The listing builds one solid part. Answer for the finished solid, in the listing's coordinates (mm). A direction names the side the tool comes from. Give positions to 0.01 mm unless a question says otherwise; leave off trailing zeros. Order: outer loops, then holes, each group sorted by start corner. A loop starts at its lowest first (then second) coordinate and runs counter-clockwise, first axis right, second up. Notation, with made-up numbers: (13.25, 38.25) - (63.25, 38.25) arc R8 cw to (63.25, 44.25) - close; hole circle Ø1 at (44, 68.5). An arc over 180 degrees is marked (long way). Answer in a Markdown table with one row per item.
from build123d import *

# Parameters (mm, degrees)
F0_R     = 25.2
F0_W     = 100
F0_H     = 15
F1_DEPTH = 15
F2_R     = 30
F5_DEPTH = 5


with BuildPart() as f1:
    # F0 (on Top) → F1 (new body)
    with BuildSketch(Plane.XY):
        with BuildLine():
            Line((-50, -85), (50, -85))
            Line((50, -85), (50, 40))
            Line((50, 40), (29.85, 40))
            ThreePointArc((29.85, 40), (0, 10.15), (-29.85, 40))
            Line((-29.85, 40), (-50, 40))
            Line((-50, 40), (-50, -85))
        make_face()
        with Locations((0, -45.2)):
            Circle(F0_R, mode=Mode.SUBTRACT)
        with BuildLine():
            Line((29.85, 40), (50, 40))
            Line((50, 40), (50, 70))
            Line((50, 70), (-50, 70))
            Line((-50, 70), (-50, 40))
            Line((-50, 40), (-29.85, 40))
            ThreePointArc((-29.85, 40), (0, 69.85), (29.85, 40))
        make_face()
        with Locations((0, 77.5)):
            Rectangle(F0_W, F0_H)
    extrude(amount=F1_DEPTH)

    # F2
    f2_edges = [f1.edges().sort_by_distance(p)[0] for p in [
        (-50, 85, 7.5),
        (50, 85, 7.5),
        (-50, -85, 7.5),
        (50, -85, 7.5),
    ]]
    fillet(f2_edges, radius=F2_R)

    # F4 (on face) → F5 (cut)
    with BuildSketch(Plane.XY.offset(15)):
        with BuildLine():
            ThreePointArc((45, 55), (37.67767, 72.67767), (20, 80))
            Line((20, 80), (-20, 80))
            ThreePointArc((-20, 80), (-37.67767, 72.67767), (-45, 55))
            Line((-45, 55), (-45, -55))
            ThreePointArc((-45, -55), (-37.67767, -72.67767), (-20, -80))
            Line((-20, -80), (20, -80))
            ThreePointArc((20, -80), (37.67767, -72.67767), (45, -55))
            Line((45, -55), (45, 55))
        make_face()
        with BuildLine():
            Line((-20, 74), (20, 74))
            ThreePointArc((20, 74), (33.435029, 68.435029), (39, 55))
            Line((39, 55), (39, -55))
            ThreePointArc((39, -55), (33.435029, -68.435029), (20, -74))
            Line((20, -74), (-20, -74))
            ThreePointArc((-20, -74), (-33.435029, -68.435029), (-39, -55))
            Line((-39, -55), (-39, 55))
            ThreePointArc((-39, 55), (-33.435029, 68.435029), (-20, 74))
        make_face(mode=Mode.SUBTRACT)
    extrude(amount=-F5_DEPTH, mode=Mode.SUBTRACT)


solid = f1.part
Item 1: Which of the six approach directions +Z, -Z, +X, -X, +Y, -Y give full straight-line access (tool end or side, diameter ignored) to faces 5 (the face through (-50, 1, 7)), 6 (the face through (33.58, -68.29, 12.54))?
Answer block:
| item | result |
|---|---|
| face 5 | +Z, -Z, -X, +Y, -Y |
| face 6 | +Z |
Item 2: Find section D-D on y = -10. Write down the section's boundary in (x, z), then the cut area to 3 significant figures.
Answer block:
| item | result |
|---|---|
| outline | (-50, 0) - (50, 0) - (50, 15) - (45, 15) - (45, 10) - (39, 10) - (39, 15) - (-39, 15) - (-39, 10) - (-45, 10) - (-45, 15) - (-50, 15) - close |
| area | 1,440 mm² |
Item 3: Find section C-C on x = 0. Write down the section's boundary in (y, z), then the cut area to 4 significant figures.
Answer block:
| item | result |
|---|---|
| outline | (-85, 0) - (-70.4, 0) - (-70.4, 15) - (-74, 15) - (-74, 10) - (-80, 10) - (-80, 15) - (-85, 15) - close; (-20, 0) - (10.15, 0) - (10.15, 15) - (-20, 15) - close; (69.85, 0) - (85, 0) - (85, 15) - (80, 15) - (80, 10) - (74, 10) - (74, 15) - (69.85, 15) - close |
| area | 838.5 mm² |
Item 4: Consider line 1 (Y direction, x = 0, z = 10.5); line 2 (Y direction, x = 0, z = 5.75); line 3 (X direction, y = 13, z = 12.75). Determine where each line is inside the solid, lowest interval first.
Answer block:
| item | result |
|---|---|
| line 1 | -85 to -80, -74 to -70.4, -20 to 10.15, 69.85 to 74, 80 to 85 |
| line 2 | -85 to -70.4, -20 to 10.15, 69.85 to 85 |
| line 3 | -50 to -45, -39 to -12.73, 12.73 to 39, 45 to 50 |
Item 5: Find section B-B on z = 8. Write down the section's boundary in (x, y).
Answer block:
| item | result |
|---|---|
| outline | (-50, -55) arc R30 ccw to (-20, -85) - (20, -85) arc R30 ccw to (50, -55) - (50, 55) arc R30 ccw to (20, 85) - (-20, 85) arc R30 ccw to (-50, 55) - close; hole circle Ø59.7 at (0, 40); hole circle Ø50.4 at (0, -45.2) |
Item 6: Find section A-A on y = 40. Write down the section's boundary in (x, z), then the cut area to 4 significant figures.
Answer block:
| item | result |
|---|---|
| outline | (-50, 0) - (-29.85, 0) - (-29.85, 15) - (-39, 15) - (-39, 10) - (-45, 10) - (-45, 15) - (-50, 15) - close; (29.85, 0) - (50, 0) - (50, 15) - (45, 15) - (45, 10) - (39, 10) - (39, 15) - (29.85, 15) - close |
| area | 544.5 mm² |
Item 7: Each of these flat-tipped pins is pushed along its axis until it touches: P1, Ø1, axis at x = -29, y = -41, coming from the -Z side; P2, Ø5, axis at x = 35.5, z = 10.5, coming from the -Y side. Where does it stop, or does it pass through?
Answer block:
| item | result |
|---|---|
| P1 | z = 0 |
| P2 | y = -82.04 |
Item 8: Determine the mould class of faces 1 (the face through (-40, 0, 10)), 2 (the face through (50, -1, 7)), 3 (the face through (-39, -1, 13)), 4 (the face through (-1, 1, 0)) for opening direction X: pulls with the +X half, pulls with the -X half, needs draft (parallel to the pull), parting line crosses it, or undercut.
Answer block:
| item | result |
|---|---|
| face 1 | undercut |
| face 2 | pulls with the +X half |
| face 3 | undercut |
| face 4 | needs draft |
